Can you work these out from the drawing? Everything is in mm from the part's minimum corner. A direction names the side the tool comes from. Coordinates: 2 decimals unless noted, no trailing zeros. Loops run counter-clockwise (first coordinate to the right, second up) from the corner with the lowest first, then second, coordinate; pieces in that order, holes last.
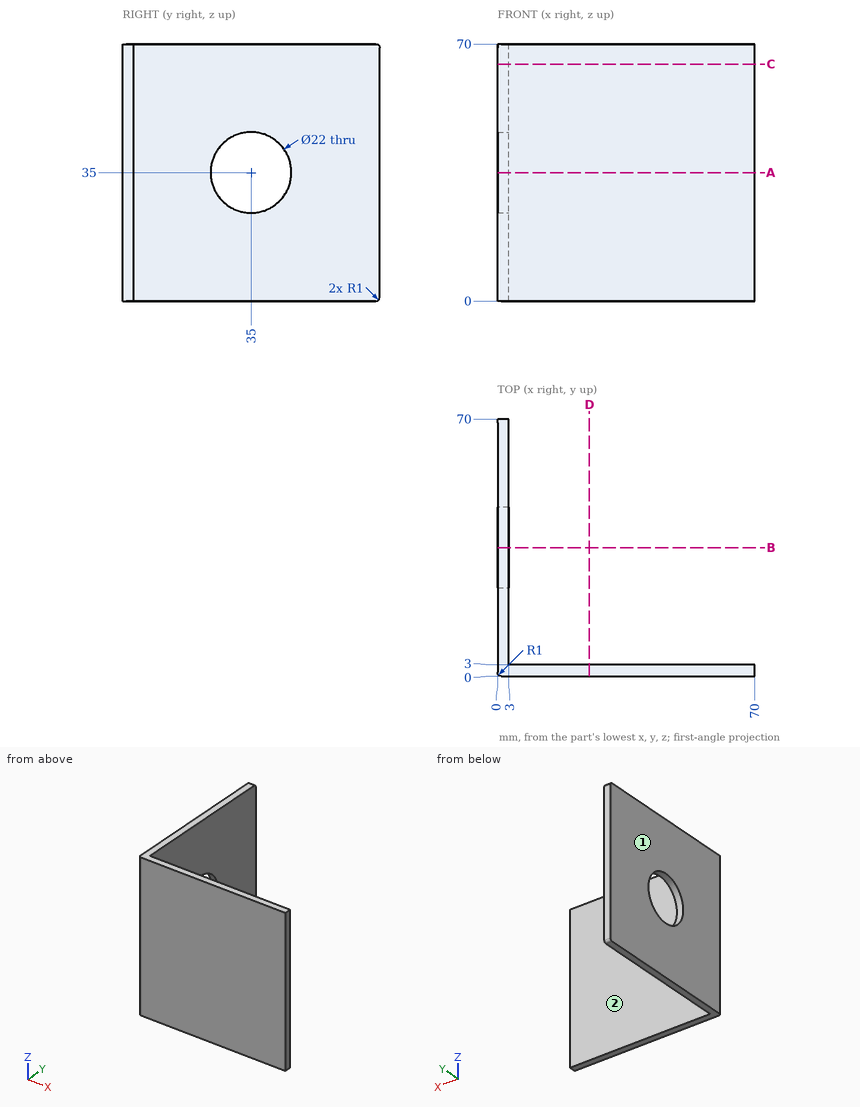
1. I want a section at C-C (z = 64.5). Please give me the cut outline in (x, y), then the cut area to 3 significant figures.
2. On a 3-axis mill with a long thin cutter (end or side, diameter ignored), from which of +Z, -Z, +X, -X, +Y, -Y can I reach the whole of each face in a straight line? I mean the marked faces 1 and 2. Say none if no direction works.
3. I want a section at D-D (x = 25). Please give me the cut outline in (y, z).
4. I need wall thicknesses on line 1 along Y through (x, z) = (5, 8.5). Which ranges of the line are inside material? Lowest first, please.
5. For pin 1 (3 mm diameter, centred on y = 58, z = 61, fed in from +X); pin 2 (10 mm diameter, centred on x = 35, z = 60, fed in from +Y), each with a flat end and sliding along its axis, tell me the tip position at first contact or that it passes through.
6. I want a section at A-A (z = 35). Please give me the cut outline in (x, y), then the cut area to 3 significant figures.
7. I want a section at B-B (y = 35). Please give me the cut outline in (x, z), then the cut area to 3 significant figures.
Response values:
1. outline: (0, 1) arc R1 ccw to (1, 0) - (70, 0) - (70, 3) - (3, 3) - (3, 70) - (0, 70) - close
1. area: 411 mm2
2. face 1: +Z, -Z, -X, +Y, -Y
2. face 2: +Z, -Z, +X, +Y
3. outline: (0, 0) - (3, 0) - (3, 70) - (0, 70) - close
4. line 1: y = 0 to 3
5. pin 1: stops at x = 3
5. pin 2: stops at y = 3
6. outline: (0, 1) arc R1 ccw to (1, 0) - (70, 0) - (70, 3) - (3, 3) - (3, 24) - (0, 24) - close; (0, 46) - (3, 46) - (3, 70) - (0, 70) - close
6. area: 345 mm2
7. outline: (0, 0) - (3, 0) - (3, 24) - (0, 24) - close; (0, 46) - (3, 46) - (3, 70) - (0, 70) - close
7. area: 144 mm2
